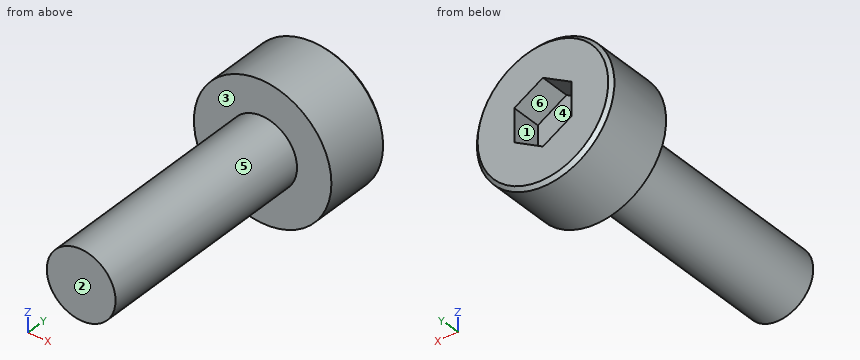
Solid Edge part; units mm, degrees
sketch "Sketch1" plane through (0, 0, 0) normal (0, -1, 0) x (1, 0, 0)
  circle A0 centre (0, 0) radius 1.5
extrude "Protrusion1" add sketch "Sketch1" against normal blind 10
sketch "Sketch2" plane through (0, 10, 0) normal (0, 1, 0) x (1, 0, 0)
  circle A0 centre (0, 0) radius 3
extrude "ExtrudedProtrusion_2" add sketch "Sketch2" along normal blind 3
sketch "Sketch3" plane through (0, 13, 0) normal (0, 1, 0) x (-1, 0, 0)
  line L0 (1.25, -0.7217) -> (1.25, 0.7217)
  line L1 (1.25, 0.7217) -> (0, 1.4434)
  line L2 (0, 1.4434) -> (-1.25, 0.7217)
  line L3 (-1.25, 0.7217) -> (-1.25, -0.7217)
  line L4 (-1.25, -0.7217) -> (0, -1.4434)
  line L5 (0, -1.4434) -> (1.25, -0.7217)
extrude "ExtrudedCutout_2" cut sketch "Sketch3" against normal blind 1.3
chamfer "Chamfer_1" distance 0.15 angle 45 1 edges at (-3, 13, 0)
properties material "Nylon, general purpose"
The model under review builds one solid part; all positions refer to its coordinate system, in mm. Face numbers are marked on the shaded views. A direction names the side the tool comes from. Give positions to 0.01 mm unless a question says otherwise; leave off trailing zeros. Order: outer loops, then holes, each group sorted by start corner. A loop starts at its lowest first (then second) coordinate and runs counter-clockwise, first axis right, second up. Notation, with made-up numbers: M 50.25,-11 L 86.25,-11 A26 ccw 86.25,24 Z; hole C 14.25,2.5 d7. An arc over 180 degrees is marked long. Use one line per item in the form item = value. Start each with the question number.
Item 1: The part is to be moulded in two halves that separate along Z. For the marked faces 3, 4, 5 and 6, say which applies: pulls with the +Z half, pulls with the -Z half, needs draft (parallel to the pull), parting line crosses it, or undercut.
Item 2: We need section A-A on z = 0. Give the boundary of the cut face in (x, y), plus the area to 3 significant figures.
Item 3: We need section B-B on y = 8.75. Give the boundary of the cut face in (x, z).
Item 4: We need section C-C on y = 11. Give the boundary of the cut face in (x, z).
Item 5: To check wall thickness, follow line 1 along Z through (x, y) = (-0.4, 4.75); line 2 along Y through (x, z) = (0.2, -1.1); line 3 along Y through (x, z) = (-2.4, 0.85). State the ranges of each line that lie inside material, in increasing order. Write a range as from..to.
Item 6: For the marked faces 1 and 2, list the 3-axis set-ups (+Z, -Z, +X, -X, +Y, -Y) from which the entire face can be reached by the end or side of a thin tool; tool diameter is ignored.
Item 7: Insertion check: pin 1 Ø1.3 at (x, z) = (-0.5, 0) entering from +Y; pin 2 Ø3 at (y, z) = (5.5, 1.5) entering from +X; pin 3 Ø1 at (x, z) = (-1.5, -0.5) entering from -Y. Each pin has a flat end and moves straight along its axis. Give the tip position at first contact, or say it passes through.
Completed:
q1.face_3 = needs draft
q1.face_4 = undercut
q1.face_5 = parting line crosses it
q1.face_6 = undercut
q2.outline = M -3,10 L -1.5,10 L -1.5,0 L 1.5,0 L 1.5,10 L 3,10 L 3,12.85 L 2.85,13 L 1.25,13 L 1.25,11.7 L -1.25,11.7 L -1.25,13 L -2.85,13 L -3,12.85 Z
q2.area = 44.7 mm²
q3.outline = C 0,0 d3
q4.outline = C 0,0 d6
q5.line_1 = -1.45..1.45
q5.line_2 = 0..11.7
q5.line_3 = 10..13
q6.face_1 = +Y
q6.face_2 = +Z, -Z, +X, -X, -Y
q7.pin_1 = 11.7
q7.pin_2 = 1.5
q7.pin_3 = 0
